Check sheet for the modelled part. Datum: model origin and axes. Units: mm. Face numbers are marked on the shaded views. A direction names the side the tool comes from. Coordinates: 2 decimals unless noted, no trailing zeros. Write each loop counter-clockwise with the first axis right and the second up, starting at its lowest first coordinate (ties: lowest second). Pieces come first, ordered by that corner, then holes. Notation, with made-up numbers: M 30,80 L 66,80 A16 cw 66,94 Z; hole C 17.25,46 d3. An arc over 180 degrees is marked long. Answer as CSV lines item,"result".
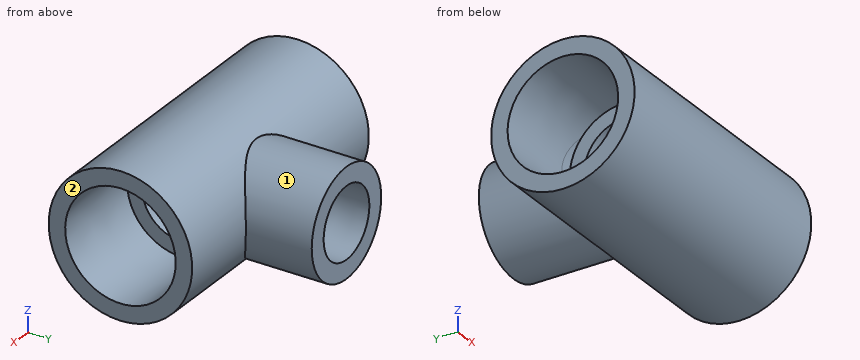
from build123d import *

# Parameters (mm, degrees)
SKETCH4_R           = 21.844
BOSS_EXTRUDE1_DEPTH = 25.4
SKETCH5_R           = 16.383
BOSS_EXTRUDE2_DEPTH = 19.05


with BuildPart() as part:
    # Sketch1 → Revolve1 (revolve)
    with BuildSketch(Plane.XY, mode=Mode.PRIVATE) as revolve1_sk:
        Polygon((-41.656, -21.844), (-12.7, -21.844), (-12.7, -16.637), (-41.656, -16.8275), align=None)
        Polygon((41.656, -16.8275), (12.7, -16.637), (12.7, -21.844), (41.656, -21.844), align=None)
    revolve(revolve1_sk.sketch.rotate(Axis((-41.656, 0, 0), (1, 0, 0)), 270), axis=Axis((-41.656, 0, 0), (1, 0, 0)))



with BuildPart() as body_2:
    # Sketch2 → Revolve2 (revolve)
    with BuildSketch(Plane.XY):
        Polygon((10.7696, 41.91), (10.6172, 19.05), (16.383, 19.05), (16.383, 41.91), align=None)
    revolve(axis=Axis((0, 0, 0), (0, 1, 0)))


with BuildPart() as part_1:
    add(part.part)

    add(body_2.part)  # Boss-Extrude1 merges body 2
    # Sketch4 → Boss-Extrude1 (add)
    with BuildSketch(Plane(origin=(-12.7, 0, 0), x_dir=(0, 0, -1), z_dir=(1, 0, 0))):
        with Locations(Location((0, 0, 0), (0, 0, 180))):
            Circle(SKETCH4_R)
    extrude(amount=BOSS_EXTRUDE1_DEPTH)

    # Sketch5 → Boss-Extrude2 (add)
    with BuildSketch(Plane.XZ.offset(-19.05)):
        Circle(SKETCH5_R)
    extrude(amount=BOSS_EXTRUDE2_DEPTH)

    # Sketch6 → Cut-Revolve1 (revolve, cut)
    with BuildSketch(Plane.XY, mode=Mode.PRIVATE) as cut_revolve1_sk:
        Polygon((-41.656, -16.8275), (-12.7, -16.637), (-12.7, -12.1539), (12.7, -12.1539), (12.7, -16.637), (41.656, -16.8275), (41.656, 0), (-41.656, 0), align=None)
    revolve(cut_revolve1_sk.sketch.rotate(Axis((41.656, 0, 0), (-1, 0, 0)), 270), axis=Axis((41.656, 0, 0), (-1, 0, 0)), mode=Mode.SUBTRACT)

    # Sketch7 → Cut-Revolve2 (revolve, cut)
    with BuildSketch(Plane.XY):
        Polygon((10.7696, 41.91), (10.6172, 19.05), (6.9342, 19.05), (6.9342, 0), (0, 0), (0, 41.91), align=None)
    revolve(axis=Axis((0, 0, 0), (0, 1, 0)), mode=Mode.SUBTRACT)


solid = part_1.part
1) Tool access check on the marked faces 1 and 2. Record the directions out of +Z, -Z, +X, -X, +Y, -Y that give a thin tool (end or side, any length) a straight path to the whole face; none if there is none.
Answer key:
face 1,"+Y"
face 2,"+Z, -Z, +X, +Y, -Y"
2) Section check D-D, the plane x = -31. Record the boundary of the cut face in (y, z), plus the area to 3 significant figures.
Answer key:
outline,"C 0,0 d43.69; hole C 0,0 d33.51"
area,"617 mm2"
3) Section check A-A, the plane x = 15. Record the boundary of the cut face in (y, z), plus the area to 3 significant figures.
Answer key:
outline,"M 20.83,-6.59 L 41.91,-6.59 L 41.91,6.59 L 20.83,6.59 A21.84 ccw long Z; hole C 0,0 d33.3"
area,"897 mm2"
4) Thickness scan on line 1 along Y through (x, z) = (7, 0); line 2 along Z through (x, y) = (0, 16.75); line 3 along X through (y, z) = (13, 0). Record the ranges inside material, lowest first.
Answer key:
line 1,"y = -21.84 to -12.15, 12.15 to 19.05"
line 2,"z = -16.38 to -6.93, 6.93 to 16.38"
line 3,"x = -12.7 to -6.93, 6.93 to 12.7"
5) Section check B-B, the plane z = 0. Give the number of separate pieces and of enclosed holes in the cut face, plus the area to 3 significant figures.
Answer key:
separate pieces,"3"
enclosed holes,"0"
area,"1,160 mm2"
6) Depth check by flat-ended pin: P1, Ø2, axis at x = -5.5, y = 3, coming from the +Z side; P2, Ø4, axis at x = -22.5, y = 17, coming from the +Z side; P3, Ø6.5, axis at x = 1.5, z = 0, coming from the +Y side. Enter the tip coordinate at first touch or a pass-through.
Answer key:
P1,"stops at z = 21.75"
P2,"stops at z = 15.88"
P3,"stops at y = -11.71"
7) Section check C-C, the plane y = 28. Record the boundary of the cut face in (x, z).
Answer key:
outline,"C 0,0 d32.77; hole C 0,0 d21.35"
